from build123d import *

# Parameters (mm, degrees)
SKETCH1_W           = 25.4
SKETCH1_H           = 50.8
SKETCH1_W_2         = 19.05
SKETCH1_H_2         = 44.45
BOSS_EXTRUDE1_DEPTH = 508
CUT_EXTRUDE1_REACH  = 513.165
SKETCH2_R           = 2.4638
CUT_EXTRUDE2_REACH  = 513.165
SKETCH3_R           = 2.4638
CUT_EXTRUDE3_REACH  = 513.165
SKETCH4_R           = 2.5796875


with BuildPart() as part:
    # Sketch1 → Boss-Extrude1 (new body)
    with BuildSketch(Plane(origin=(0, 0, 0), x_dir=(1, 0, 0), z_dir=(0, 1, 0))):
        with Locations((12.7, 25.4)):
            Rectangle(SKETCH1_W, SKETCH1_H)
        with Locations((12.7, 25.4)):
            Rectangle(SKETCH1_W_2, SKETCH1_H_2, mode=Mode.SUBTRACT)
    extrude(amount=BOSS_EXTRUDE1_DEPTH)

    # Sketch2 → Cut-Extrude1 (cut, up to next)
    with BuildSketch(Plane(origin=(0, 0, -50.8), x_dir=(-1, 0, 0), z_dir=(0, 0, -1)), mode=Mode.PRIVATE) as cut_extrude1_sk1:
        with Locations((-12.7, 12.7)):
            Circle(SKETCH2_R)
    cut_extrude1_tool1 = extrude(cut_extrude1_sk1.sketch, amount=-CUT_EXTRUDE1_REACH, mode=Mode.PRIVATE) & part.part
    # Sketch2 → Cut-Extrude1 (cut, up to next)
    with BuildSketch(Plane(origin=(0, 0, -50.8), x_dir=(-1, 0, 0), z_dir=(0, 0, -1)), mode=Mode.PRIVATE) as cut_extrude1_sk2:
        with Locations((-12.7, 50.8)):
            Circle(SKETCH2_R)
    cut_extrude1_tool2 = extrude(cut_extrude1_sk2.sketch, amount=-CUT_EXTRUDE1_REACH, mode=Mode.PRIVATE) & part.part
    # Sketch2 → Cut-Extrude1 (cut, up to next)
    with BuildSketch(Plane(origin=(0, 0, -50.8), x_dir=(-1, 0, 0), z_dir=(0, 0, -1)), mode=Mode.PRIVATE) as cut_extrude1_sk3:
        with Locations((-12.7, 177.8)):
            Circle(SKETCH2_R)
    cut_extrude1_tool3 = extrude(cut_extrude1_sk3.sketch, amount=-CUT_EXTRUDE1_REACH, mode=Mode.PRIVATE) & part.part
    # Sketch2 → Cut-Extrude1 (cut, up to next)
    with BuildSketch(Plane(origin=(0, 0, -50.8), x_dir=(-1, 0, 0), z_dir=(0, 0, -1)), mode=Mode.PRIVATE) as cut_extrude1_sk4:
        with Locations((-12.7, 215.9)):
            Circle(SKETCH2_R)
    cut_extrude1_tool4 = extrude(cut_extrude1_sk4.sketch, amount=-CUT_EXTRUDE1_REACH, mode=Mode.PRIVATE) & part.part
    # Sketch2 → Cut-Extrude1 (cut, up to next)
    with BuildSketch(Plane(origin=(0, 0, -50.8), x_dir=(-1, 0, 0), z_dir=(0, 0, -1)), mode=Mode.PRIVATE) as cut_extrude1_sk5:
        with Locations((-12.7, 241.3)):
            Circle(SKETCH2_R)
    cut_extrude1_tool5 = extrude(cut_extrude1_sk5.sketch, amount=-CUT_EXTRUDE1_REACH, mode=Mode.PRIVATE) & part.part
    # Sketch2 → Cut-Extrude1 (cut, up to next)
    with BuildSketch(Plane(origin=(0, 0, -50.8), x_dir=(-1, 0, 0), z_dir=(0, 0, -1)), mode=Mode.PRIVATE) as cut_extrude1_sk6:
        with Locations((-12.7, 266.7)):
            Circle(SKETCH2_R)
    cut_extrude1_tool6 = extrude(cut_extrude1_sk6.sketch, amount=-CUT_EXTRUDE1_REACH, mode=Mode.PRIVATE) & part.part
    # Sketch2 → Cut-Extrude1 (cut, up to next)
    with BuildSketch(Plane(origin=(0, 0, -50.8), x_dir=(-1, 0, 0), z_dir=(0, 0, -1)), mode=Mode.PRIVATE) as cut_extrude1_sk7:
        with Locations((-12.7, 292.1)):
            Circle(SKETCH2_R)
    cut_extrude1_tool7 = extrude(cut_extrude1_sk7.sketch, amount=-CUT_EXTRUDE1_REACH, mode=Mode.PRIVATE) & part.part
    # Sketch2 → Cut-Extrude1 (cut, up to next)
    with BuildSketch(Plane(origin=(0, 0, -50.8), x_dir=(-1, 0, 0), z_dir=(0, 0, -1)), mode=Mode.PRIVATE) as cut_extrude1_sk8:
        with Locations((-12.7, 330.2)):
            Circle(SKETCH2_R)
    cut_extrude1_tool8 = extrude(cut_extrude1_sk8.sketch, amount=-CUT_EXTRUDE1_REACH, mode=Mode.PRIVATE) & part.part
    # Sketch2 → Cut-Extrude1 (cut, up to next)
    with BuildSketch(Plane(origin=(0, 0, -50.8), x_dir=(-1, 0, 0), z_dir=(0, 0, -1)), mode=Mode.PRIVATE) as cut_extrude1_sk9:
        with Locations((-12.7, 457.2)):
            Circle(SKETCH2_R)
    cut_extrude1_tool9 = extrude(cut_extrude1_sk9.sketch, amount=-CUT_EXTRUDE1_REACH, mode=Mode.PRIVATE) & part.part
    # Sketch2 → Cut-Extrude1 (cut, up to next)
    with BuildSketch(Plane(origin=(0, 0, -50.8), x_dir=(-1, 0, 0), z_dir=(0, 0, -1)), mode=Mode.PRIVATE) as cut_extrude1_sk10:
        with Locations((-12.7, 495.3)):
            Circle(SKETCH2_R)
    cut_extrude1_tool10 = extrude(cut_extrude1_sk10.sketch, amount=-CUT_EXTRUDE1_REACH, mode=Mode.PRIVATE) & part.part
    add(cut_extrude1_tool1.solids().sort_by_distance((12.7, 12.7, -50.8))[0], mode=Mode.SUBTRACT)
    add(cut_extrude1_tool2.solids().sort_by_distance((12.7, 50.8, -50.8))[0], mode=Mode.SUBTRACT)
    add(cut_extrude1_tool3.solids().sort_by_distance((12.7, 177.8, -50.8))[0], mode=Mode.SUBTRACT)
    add(cut_extrude1_tool4.solids().sort_by_distance((12.7, 215.9, -50.8))[0], mode=Mode.SUBTRACT)
    add(cut_extrude1_tool5.solids().sort_by_distance((12.7, 241.3, -50.8))[0], mode=Mode.SUBTRACT)
    add(cut_extrude1_tool6.solids().sort_by_distance((12.7, 266.7, -50.8))[0], mode=Mode.SUBTRACT)
    add(cut_extrude1_tool7.solids().sort_by_distance((12.7, 292.1, -50.8))[0], mode=Mode.SUBTRACT)
    add(cut_extrude1_tool8.solids().sort_by_distance((12.7, 330.2, -50.8))[0], mode=Mode.SUBTRACT)
    add(cut_extrude1_tool9.solids().sort_by_distance((12.7, 457.2, -50.8))[0], mode=Mode.SUBTRACT)
    add(cut_extrude1_tool10.solids().sort_by_distance((12.7, 495.3, -50.8))[0], mode=Mode.SUBTRACT)

    # Sketch3 → Cut-Extrude2 (cut, up to next)
    with BuildSketch(Plane.XY, mode=Mode.PRIVATE) as cut_extrude2_sk1:
        with Locations((12.7, 63.5)):
            Circle(SKETCH3_R)
    cut_extrude2_tool1 = extrude(cut_extrude2_sk1.sketch, amount=-CUT_EXTRUDE2_REACH, mode=Mode.PRIVATE) & part.part
    # Sketch3 → Cut-Extrude2 (cut, up to next)
    with BuildSketch(Plane.XY, mode=Mode.PRIVATE) as cut_extrude2_sk2:
        with Locations((12.7, 139.7)):
            Circle(SKETCH3_R)
    cut_extrude2_tool2 = extrude(cut_extrude2_sk2.sketch, amount=-CUT_EXTRUDE2_REACH, mode=Mode.PRIVATE) & part.part
    # Sketch3 → Cut-Extrude2 (cut, up to next)
    with BuildSketch(Plane.XY, mode=Mode.PRIVATE) as cut_extrude2_sk3:
        with Locations(Location((12.7, 215.9, 0), (0, 0, 180))):
            Circle(SKETCH3_R)
    cut_extrude2_tool3 = extrude(cut_extrude2_sk3.sketch, amount=-CUT_EXTRUDE2_REACH, mode=Mode.PRIVATE) & part.part
    # Sketch3 → Cut-Extrude2 (cut, up to next)
    with BuildSketch(Plane.XY, mode=Mode.PRIVATE) as cut_extrude2_sk4:
        with Locations(Location((12.7, 292.1, 0), (0, 0, 180))):
            Circle(SKETCH3_R)
    cut_extrude2_tool4 = extrude(cut_extrude2_sk4.sketch, amount=-CUT_EXTRUDE2_REACH, mode=Mode.PRIVATE) & part.part
    # Sketch3 → Cut-Extrude2 (cut, up to next)
    with BuildSketch(Plane.XY, mode=Mode.PRIVATE) as cut_extrude2_sk5:
        with Locations((12.7, 368.3)):
            Circle(SKETCH3_R)
    cut_extrude2_tool5 = extrude(cut_extrude2_sk5.sketch, amount=-CUT_EXTRUDE2_REACH, mode=Mode.PRIVATE) & part.part
    # Sketch3 → Cut-Extrude2 (cut, up to next)
    with BuildSketch(Plane.XY, mode=Mode.PRIVATE) as cut_extrude2_sk6:
        with Locations((12.7, 444.5)):
            Circle(SKETCH3_R)
    cut_extrude2_tool6 = extrude(cut_extrude2_sk6.sketch, amount=-CUT_EXTRUDE2_REACH, mode=Mode.PRIVATE) & part.part
    add(cut_extrude2_tool1.solids().sort_by_distance((12.7, 63.5, 0))[0], mode=Mode.SUBTRACT)
    add(cut_extrude2_tool2.solids().sort_by_distance((12.7, 139.7, 0))[0], mode=Mode.SUBTRACT)
    add(cut_extrude2_tool3.solids().sort_by_distance((12.7, 215.9, 0))[0], mode=Mode.SUBTRACT)
    add(cut_extrude2_tool4.solids().sort_by_distance((12.7, 292.1, 0))[0], mode=Mode.SUBTRACT)
    add(cut_extrude2_tool5.solids().sort_by_distance((12.7, 368.3, 0))[0], mode=Mode.SUBTRACT)
    add(cut_extrude2_tool6.solids().sort_by_distance((12.7, 444.5, 0))[0], mode=Mode.SUBTRACT)

    # Sketch4 → Cut-Extrude3 (cut, up to next)
    with BuildSketch(Plane.ZY, mode=Mode.PRIVATE) as cut_extrude3_sk1:
        with Locations((-38.110518668, 96.635101662)):
            Circle(SKETCH4_R)
    cut_extrude3_tool1 = extrude(cut_extrude3_sk1.sketch, amount=-CUT_EXTRUDE3_REACH, mode=Mode.PRIVATE) & part.part
    # Sketch4 → Cut-Extrude3 (cut, up to next)
    with BuildSketch(Plane.ZY, mode=Mode.PRIVATE) as cut_extrude3_sk2:
        with Locations((-38.110518668, 411.364898332)):
            Circle(SKETCH4_R)
    cut_extrude3_tool2 = extrude(cut_extrude3_sk2.sketch, amount=-CUT_EXTRUDE3_REACH, mode=Mode.PRIVATE) & part.part
    # Sketch4 → Cut-Extrude3 (cut, up to next)
    with BuildSketch(Plane.ZY, mode=Mode.PRIVATE) as cut_extrude3_sk3:
        with Locations((-12.710518668, 411.364898332)):
            Circle(SKETCH4_R)
    cut_extrude3_tool3 = extrude(cut_extrude3_sk3.sketch, amount=-CUT_EXTRUDE3_REACH, mode=Mode.PRIVATE) & part.part
    # Sketch4 → Cut-Extrude3 (cut, up to next)
    with BuildSketch(Plane.ZY, mode=Mode.PRIVATE) as cut_extrude3_sk4:
        with Locations((-12.710518668, 96.635101662)):
            Circle(SKETCH4_R)
    cut_extrude3_tool4 = extrude(cut_extrude3_sk4.sketch, amount=-CUT_EXTRUDE3_REACH, mode=Mode.PRIVATE) & part.part
    add(cut_extrude3_tool1.solids().sort_by_distance((0, 96.635102, -38.110519))[0], mode=Mode.SUBTRACT)
    add(cut_extrude3_tool2.solids().sort_by_distance((0, 411.364898, -38.110519))[0], mode=Mode.SUBTRACT)
    add(cut_extrude3_tool3.solids().sort_by_distance((0, 411.364898, -12.710519))[0], mode=Mode.SUBTRACT)
    add(cut_extrude3_tool4.solids().sort_by_distance((0, 96.635102, -12.710519))[0], mode=Mode.SUBTRACT)


solid = part.part
Part model, mm, in its own coordinate system. A direction names the side the tool comes from. Coordinates: 2 decimals unless noted, no trailing zeros. Loops run counter-clockwise (first coordinate to the right, second up) from the corner with the lowest first, then second, coordinate; pieces in that order, holes last. Notation, with made-up numbers: (-37, 82.5) -> (-13, 82.5) arc R14 cw to (-13, 93.5) -> close; hole circle Ø6 at (20.25, 44). An arc over 180 degrees is marked (long way). Use a Markdown table: item, result. Add a question column.
Item 1: Flat gauge pins, fed straight in: P1, Ø4, axis at x = 12.7, y = 215.9, coming from the +Z side; P2, Ø4.5, axis at x = 12.7, y = 63.5, coming from the +Z side (3 decimals); P3, Ø4.5, axis at x = 12.7, y = 330.2, coming from the -Z side (3 decimals). Where does each tip first touch, or does it go through?
Item 2: Band-saw the part on A-A on z = -29.5. Write the cut outline in (x, y) (3 decimals).
Item 3: Band-saw the part on B-B on y = 420. Write the cut outline in (x, z) (3 decimals).
Item 4: Which spindle directions (+Z, -Z, +X, -X, +Y, -Y) get a long thin tool onto all of the face, cutting with end or side? Do faces 4 (the flat face through (13, 250, -47.625)), 5 (the flat face through (2, 508, -24)). Say none if no direction does.
Item 5: Probe probe 1 along Z at (x, y) = (13, 427.5) (3 decimals); probe 2 along X at (y, z) = (448, -47.5) (3 decimals); probe 3 along X at (y, z) = (215.9, -49.1). List the from-to ranges inside material, lowest first.
Item 6: Pull direction X, two halves, no side cores. Call faces 1 (the flat face through (25.4, 250, -25)), 2 (the flat face through (3.175, 250, -25)), 3 (the flat face through (0, 250, -25)): +X half, -X half, draft (parallel to the pull), parting line (faces both ways), or undercut.
Geometry says:
| question | item | result |
|---|---|---|
| 1 | P1 | through |
| 1 | P2 | z = -47.625 |
| 1 | P3 | z = -3.175 |
| 2 | outline | (0, 0) -> (3.175, 0) -> (3.175, 508) -> (0, 508) -> close; (22.225, 0) -> (25.4, 0) -> (25.4, 508) -> (22.225, 508) -> close |
| 3 | outline | (0, -50.8) -> (25.4, -50.8) -> (25.4, 0) -> (0, 0) -> close; hole (3.175, -47.625) -> (22.225, -47.625) -> (22.225, -3.175) -> (3.175, -3.175) -> close |
| 4 | face 4 | +Y, -Y |
| 4 | face 5 | +Z, -Z, +X, -X, +Y |
| 5 | probe 1 | -50.8 to -47.625, -3.175 to 0 |
| 5 | probe 2 | 0 to 3.175, 22.225 to 25.4 |
| 5 | probe 3 | 0 to 10.24, 15.16 to 25.4 |
| 6 | face 1 | +X half |
| 6 | face 2 | undercut |
| 6 | face 3 | -X half |
